For this review, use the dimensioned drawing (mm, ordinates from the lowest corner) and the shaded views. A direction names the side the tool comes from. Give positions to 0.01 mm unless a question says otherwise; leave off trailing zeros. Loops run counter-clockwise (first coordinate to the right, second up) from the corner with the lowest first, then second, coordinate; pieces in that order, holes last. Notation, with made-up numbers: (44.25, 88.5) -> (77.25, 88.5) arc R20 cw to (77.25, 105.5) -> close; hole circle Ø5 at (-38.75, 88.5). An arc over 180 degrees is marked (long way). Write each question's results on one line, items separated by ' | '. Start each with the question number.
Q1. Insertion check: pin 1 Ø1.5 at (x, z) = (43, 33) entering from +Y; pin 2 Ø8 at (x, y) = (49, 8.5) entering from -Z; pin 3 Ø1.5 at (x, y) = (24.5, 22) entering from -Z; pin 4 Ø11 at (x, z) = (23, 18.5) entering from -Y. Each pin has a flat end and moves straight along its axis. Give the tip position at first contact, or say it passes through.
Q2. We need section C-C (z = 19). Write out the cut boundary in (x, y), plus the area to 3 significant figures.
Q3. Machinability: for the marked faces 5 and 6, which of the approach directions +Z, -Z, +X, -X, +Y, -Y give a long, thin tool a straight path to every point of the face, cutting with its end or side? Answer none if there is none.
Q4. We need section D-D (y = 3). Write out the cut boundary in (x, z) (3 decimals).
Q5. Wall thickness on L1, parallel to Z at x = 34, y = 8; L2, parallel to Y at x = 34.5, z = 20.5; L3, parallel to Y at x = 49, z = 33.2: over which ranges is each line inside the solid? List them lowest first. Write a range as [from, to].
Q6. We need section A-A (x = 24.5). Write out the cut boundary in (y, z).
Q7. Mouldability with a two-part tool opening along Z and no side actions: class the marked faces 1, 2, 3 and 4 as released by +Z, released by -Z, zero draft, split by the parting line, or undercut.
Q8. We need section B-B (y = 10). Write out the cut boundary in (x, z).
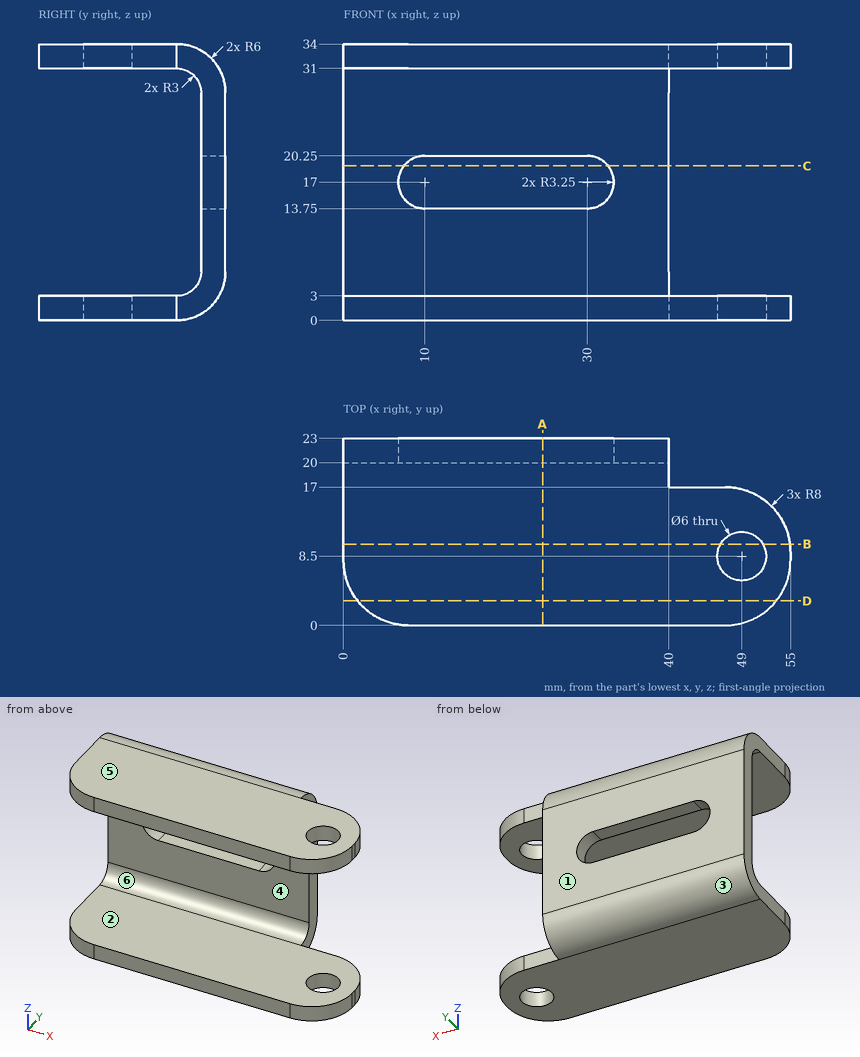
Output:
1) pin 1: y = 17 | pin 2: z = 0 | pin 3: z = 1.76 | pin 4: y = 20
2) outline: (0, 20) -> (7.44, 20) -> (7.44, 23) -> (0, 23) -> close; (32.56, 20) -> (40, 20) -> (40, 23) -> (32.56, 23) -> close | area: 44.6 mm2
3) face 5: +Z, +X, -X, +Y, -Y | face 6: +X, -X, -Y
4) outline: (1.755, 0) -> (53.245, 0) -> (53.245, 3) -> (1.755, 3) -> close; (1.755, 31) -> (53.245, 31) -> (53.245, 34) -> (1.755, 34) -> close
5) L1: [0, 3], [31, 34] | L2: [20, 23] | L3: [0.25, 5.5], [11.5, 16.75]
6) outline: (0, 0) -> (17, 0) arc R6 ccw to (23, 6) -> (23, 13.75) -> (20, 13.75) -> (20, 6) arc R3 cw to (17, 3) -> (0, 3) -> close; (0, 31) -> (17, 31) arc R3 cw to (20, 28) -> (20, 20.25) -> (23, 20.25) -> (23, 28) arc R6 ccw to (17, 34) -> (0, 34) -> close
7) face 1: zero draft | face 2: undercut | face 3: released by -Z | face 4: undercut
8) outline: (0, 0) -> (46.4, 0) -> (46.4, 3) -> (0, 3) -> close; (0, 31) -> (46.4, 31) -> (46.4, 34) -> (0, 34) -> close; (51.6, 0) -> (54.94, 0) -> (54.94, 3) -> (51.6, 3) -> close; (51.6, 31) -> (54.94, 31) -> (54.94, 34) -> (51.6, 34) -> close
